from build123d import *

# Parameters (mm, degrees)
F0_W     = 381
F0_H     = 127
F1_DEPTH = 50.8
F2_W     = 26.67
F2_H     = 114.3
F2_W_2   = 38.1
F3_DEPTH = 44.45
F4_W     = 76.2
F4_H     = 114.3
F4_W_2   = 200.66
F5_DEPTH = 34.29
F6_R     = 3.175
F7_DEPTH = 16.511


with BuildPart() as f1:
    # F0 (on Front) → F1 (new body)
    with BuildSketch(Plane.XZ):
        with Locations((190.5, 63.5)):
            Rectangle(F0_W, F0_H)
    extrude(amount=F1_DEPTH)

    # F2 (on face) → F3 (cut)
    with BuildSketch(Plane.XZ.offset(50.8)):
        with Locations((19.685, 63.5)):
            Rectangle(F2_W, F2_H)
        with Locations((128.27, 63.5)):
            Rectangle(F2_W_2, F2_H)
        with Locations((361.315, 63.5)):
            Rectangle(F2_W, F2_H)
    extrude(amount=-F3_DEPTH, mode=Mode.SUBTRACT)

    # F4 (on face) → F5 (cut)
    with BuildSketch(Plane.XZ.offset(50.8)):
        with Locations((71.12, 63.5)):
            Rectangle(F4_W, F4_H)
        with Locations((247.65, 63.5)):
            Rectangle(F4_W_2, F4_H)
    extrude(amount=-F5_DEPTH, mode=Mode.SUBTRACT)

    # F6 (on face) → F7 (cut, through all)
    with BuildSketch(Plane.XZ.offset(16.51)):
        with Locations((69.52478, 63.5)):
            Circle(F6_R)
        with Locations((316.042095, 63.5)):
            Circle(F6_R)
    extrude(amount=-F7_DEPTH, mode=Mode.SUBTRACT)


solid = f1.part
Work out the finished part from the listing and answer in its coordinate system (mm). A direction names the side the tool comes from. Coordinates: 2 decimals unless noted, no trailing zeros. Write each loop counter-clockwise with the first axis right and the second up, starting at its lowest first coordinate (ties: lowest second). Pieces come first, ordered by that corner, then holes. Notation, with made-up numbers: (28.25, 88) - (73.25, 88) arc R23 ccw to (73.25, 106) - close; hole circle Ø3 at (19, -7.5). An arc over 180 degrees is marked (long way). One line per question, with ' | ' between items.
1) Consider probe 1 along X at (y, z) = (-12, 63); probe 2 along X at (y, z) = (-11, 7); probe 3 along X at (y, z) = (-46, 14). Determine where each line is inside the solid, lowest interval first. Write a range as [from, to].
Checks:
probe 1: [0, 6.35], [33.02, 66.39], [72.66, 109.22], [147.32, 312.91], [319.18, 347.98], [374.65, 381] | probe 2: [0, 6.35], [33.02, 109.22], [147.32, 347.98], [374.65, 381] | probe 3: [0, 6.35], [374.65, 381]
2) Flat-ended cylindrical pins translate along their axes: P1, Ø21.5, axis at x = 362.5, z = 78.5, coming from the -Y side; P2, Ø2, axis at y = -26, z = 32, coming from the -X side; P3, Ø4, axis at x = 69.52, z = 63.5, coming from the +Y side; P4, Ø21.5, axis at x = 23, z = 58.5, coming from the -Y side. Find the tip coordinate at first contact, or state that the pin passes through.
Checks:
P1: y = -6.35 | P2: x = 0 | P3: through | P4: y = -16.51
3) Find section B-B, the plane z = 95.5. Determine the outline of the cut face in (x, y), and give its area (3 significant figures).
Checks:
outline: (0, -50.8) - (6.35, -50.8) - (6.35, -6.35) - (33.02, -6.35) - (33.02, -16.51) - (109.22, -16.51) - (109.22, -6.35) - (147.32, -6.35) - (147.32, -16.51) - (347.98, -16.51) - (347.98, -6.35) - (374.65, -6.35) - (374.65, -50.8) - (381, -50.8) - (381, 0) - (0, 0) - close | area: 5,800 mm2
4) The mould has two halves that part along Z. Classify faces 3 (the face through (188, -25, 0)), 4 (the face through (361, -6.35, 64)), 5 (the face through (19, -6.35, 64)), 6 (the face through (0, -25, 63)): +Z half, -Z half, draft (parallel to the pull), parting line (faces both ways), or undercut.
Checks:
face 3: -Z half | face 4: undercut | face 5: undercut | face 6: draft
5) Find section A-A, the plane y = -13. Determine the outline of the cut face in (x, z) (3 decimals).
Checks:
outline: (0, 0) - (381, 0) - (381, 127) - (0, 127) - close; hole (6.35, 6.35) - (33.02, 6.35) - (33.02, 120.65) - (6.35, 120.65) - close; hole circle Ø6.35 at (69.525, 63.5); hole (109.22, 6.35) - (147.32, 6.35) - (147.32, 120.65) - (109.22, 120.65) - close; hole circle Ø6.35 at (316.042, 63.5); hole (347.98, 6.35) - (374.65, 6.35) - (374.65, 120.65) - (347.98, 120.65) - close
6) Find section D-D, the plane y = -37. Determine the outline of the cut face in (x, z).
Checks:
outline: (0, 0) - (381, 0) - (381, 127) - (0, 127) - close; hole (6.35, 6.35) - (374.65, 6.35) - (374.65, 120.65) - (6.35, 120.65) - close
7) Find section C-C, the plane x = 279. Determine the outline of the cut face in (y, z), and give its area (3 significant figures).
Checks:
outline: (-50.8, 0) - (0, 0) - (0, 127) - (-50.8, 127) - (-50.8, 120.65) - (-16.51, 120.65) - (-16.51, 6.35) - (-50.8, 6.35) - close | area: 2,530 mm2
8) For faces 1 (the face through (319.07, -8.37, 64.45)), 2 (the face through (246, -16.51, 64)), determine the directions among +Z, -Z, +X, -X, +Y, -Y from which every point of the face is accessible in a straight line to the end or side of a thin tool.
Checks:
face 1: +Y, -Y | face 2: -Y
